Geometry: final body of the model. Coordinates: model frame, mm. A direction names the side the tool comes from. Coordinates: 2 decimals unless noted, no trailing zeros. Loops run counter-clockwise (first coordinate to the right, second up) from the corner with the lowest first, then second, coordinate; pieces in that order, holes last. Notation, with made-up numbers: (-12.75, -17) -> (8.25, -17) arc R13 ccw to (8.25, -1) -> close; hole circle Ø2 at (83, -6). An arc over 180 degrees is marked (long way). One line per item, written item: value. Start each with the question number.
Item 1: Section query C-C on x = -10.5. Return loops of the section in (y, z).
Item 2: Section query B-B on z = 0. Return loops of the section in (x, y) (3 decimals), then the cut area to 3 significant figures.
Item 3: Mould query, pull axis Z, two halves, no side actions, for faces 3 (the flat face through (-6, 1.3, -2)), 4 (the flat face through (16.25, 4, 0)), 5 (the flat face through (0, 4, 8.25)). Classes: +Z half, -Z half, draft (parallel to the pull), parting line (faces both ways), or undercut.
Item 4: Section query A-A on y = 1.75. Return loops of the section in (x, z) (3 decimals), then the cut area to 3 significant figures.
Item 5: Contact query for a flat-ended pin moving along its axis: pin 1 Ø4 at (x, z) = (0, 0) entering from -Y. Output: stop coordinate, or through.
Item 6: Set-up query: faces 1 (the flat face through (0, 4, -8.25)), 2 (the cylindrical face through (-4.1, 0.6, -5.3)). Return all of +Z, -Z, +X, -X, +Y, -Y with unobstructed straight access to the full face (end or side cutting, diameter ignored); none if empty.
Item 7: Ray query, probe 1 along X at (y, z) = (2.45, 0) (3 decimals); probe 2 along X at (y, z) = (0.65, 0); probe 3 along Y at (x, z) = (-1, 3.25). Return the intervals inside material, ascending. Write a range as from..to.
Item 8: Section query D-D on x = 0. Return loops of the section in (y, z) (3 decimals).
from build123d import *

# Parameters (mm, degrees)
SKETCH1_R           = 6.7
SKETCH1_R_2         = 6.055
BOSS_EXTRUDE1_DEPTH = 1.3
SKETCH1_2_R         = 6.055
BOSS_EXTRUDE2_DEPTH = 5.6
SKETCH2_W           = 32.5
SKETCH2_H           = 16.5
BOSS_EXTRUDE3_DEPTH = 11
FILLET1_R           = 3


with BuildPart() as part:
    # Sketch1 → Boss-Extrude1 (new body)
    with BuildSketch(Plane(origin=(0, 0, 0), x_dir=(1, 0, 0), z_dir=(0, 1, 0))):
        with Locations(Location((0, 0, 0), (0, 0, 270))):
            Circle(SKETCH1_R)
        with Locations(Location((0, 0, 0), (0, 0, 270))):
            Circle(SKETCH1_R_2, mode=Mode.SUBTRACT)
    extrude(amount=BOSS_EXTRUDE1_DEPTH)

    # Sketch1_2 → Boss-Extrude2 (add)
    with BuildSketch(Plane(origin=(0, 0, 0), x_dir=(1, 0, 0), z_dir=(0, 1, 0))):
        with Locations(Location((0, 0, 0), (0, 0, 270))):
            Circle(SKETCH1_2_R)
    extrude(amount=BOSS_EXTRUDE2_DEPTH)


with BuildPart() as body_2:
    # Sketch2 → Boss-Extrude3 (new body)
    with BuildSketch(Plane(origin=(0, 0, 0), x_dir=(1, 0, 0), z_dir=(0, 1, 0))):
        Rectangle(SKETCH2_W, SKETCH2_H)
    extrude(amount=BOSS_EXTRUDE3_DEPTH)

    # Combine1: cut part
    add(part.part, mode=Mode.SUBTRACT)

    # Fillet1
    fillet1_edges = [body_2.edges().sort_by_distance(p)[0] for p in [
        (-16.25, 11, 0),
        (0, 11, 8.25),
        (16.25, 11, 0),
        (0, 11, -8.25),
    ]]
    fillet(fillet1_edges, radius=FILLET1_R)


solid = body_2.part
Reply:
1. outline: (0, -8.25) -> (8, -8.25) arc R3 ccw to (11, -5.25) -> (11, 5.25) arc R3 ccw to (8, 8.25) -> (0, 8.25) -> close
2. outline: (-16.25, 0) -> (-6.7, 0) -> (-6.7, 1.3) -> (-6.055, 1.3) -> (-6.055, 5.6) -> (6.055, 5.6) -> (6.055, 1.3) -> (6.7, 1.3) -> (6.7, 0) -> (16.25, 0) -> (16.25, 8) arc R3 ccw to (13.25, 11) -> (-13.25, 11) arc R3 ccw to (-16.25, 8) -> close
2. area: 284 mm²
3. face 3: undercut
3. face 4: draft
3. face 5: +Z half
4. outline: (-16.25, -8.25) -> (16.25, -8.25) -> (16.25, 8.25) -> (-16.25, 8.25) -> close; hole circle Ø12.11 at (0, 0)
4. area: 421 mm²
5. pin 1: stops at y = 5.6
6. face 1: -Z, +X, -X, +Y, -Y
6. face 2: -Y
7. probe 1: x = -16.25..-6.055, 6.055..16.25
7. probe 2: x = -16.25..-6.7, 6.7..16.25
7. probe 3: y = 5.6..11
8. outline: (0, -8.25) -> (8, -8.25) arc R3 ccw to (11, -5.25) -> (11, 5.25) arc R3 ccw to (8, 8.25) -> (0, 8.25) -> (0, 6.7) -> (1.3, 6.7) -> (1.3, 6.055) -> (5.6, 6.055) -> (5.6, -6.055) -> (1.3, -6.055) -> (1.3, -6.7) -> (0, -6.7) -> close
